```python
from build123d import *

# Parameters (mm, degrees)
SKETCH1_R           = 2.2
SKETCH1_R_2         = 0.75
BOSS_EXTRUDE1_DEPTH = 4.5
SKETCH1_3_R         = 0.75
BOSS_EXTRUDE2_DEPTH = 30


with BuildPart() as part:
    # Sketch1 → Boss-Extrude1 (new body)
    with BuildSketch(Plane(origin=(-110.040337845, 0, 0), x_dir=(0, 0, -1), z_dir=(1, 0, 0))):
        with BuildLine():
            Line((219.791431391, 54.406766631), (219.791431391, 56.131766631))
            ThreePointArc((219.791431391, 56.131766631), (219.498538172, 56.838873413), (218.791431391, 57.131766631))
            Line((218.791431391, 57.131766631), (213.191431391, 57.131766631))
            Line((213.191431391, 57.131766631), (213.191431391, 48.731766631))
            Line((213.191431391, 48.731766631), (219.791431391, 48.731766631))
            Line((219.791431391, 48.731766631), (219.791431391, 52.056766631))
            Line((219.791431391, 52.056766631), (219.351370906, 52.056766631))
            ThreePointArc((219.351370906, 52.056766631), (215.291431391, 53.231766631), (219.351370906, 54.406766631))
            Line((219.351370906, 54.406766631), (219.791431391, 54.406766631))
        make_face()
        with BuildLine():
            Line((219.791431391, 48.731766631), (213.191431391, 48.731766631))
            Line((213.191431391, 48.731766631), (213.191431391, 38.831766631))
            Line((213.191431391, 38.831766631), (218.291431391, 38.831766631))
            ThreePointArc((218.291431391, 38.831766631), (219.352091563, 39.27110646), (219.791431391, 40.331766631))
            Line((219.791431391, 40.331766631), (219.791431391, 48.731766631))
        make_face()
        with Locations((217.491431391, 42.731766631)):
            Circle(SKETCH1_R, mode=Mode.SUBTRACT)
        with BuildLine():
            Line((162.791431391, 64.577419509), (162.791431391, 55.557459873))
            ThreePointArc((162.791431391, 55.557459873), (163.541431391, 56.307459873), (164.291431391, 55.557459873))
            ThreePointArc((164.291431391, 55.557459873), (164.071761481, 55.027129792), (163.541431403, 54.807459873))
            Line((163.541431403, 54.807459873), (165.491431391, 54.807459873))
            Line((165.491431391, 54.807459873), (165.491431391, 57.431766631))
            Line((165.491431391, 57.431766631), (172.391431391, 57.431766631))
            Line((172.391431391, 57.431766631), (172.391431391, 58.231766631))
            Line((172.391431391, 58.231766631), (213.191431391, 58.231766631))
            Line((213.191431391, 58.231766631), (213.191431391, 57.431766631))
            Line((213.191431391, 57.431766631), (219.791431391, 57.431766631))
            Line((219.791431391, 57.431766631), (219.791431391, 60.200456158))
            Line((219.791431391, 60.200456158), (162.791431391, 64.577419509))
        make_face()
        with BuildLine():
            Line((219.791431391, 56.131766631), (219.791431391, 57.431766631))
            Line((219.791431391, 57.431766631), (213.191431391, 57.431766631))
            Line((213.191431391, 57.431766631), (213.191431391, 57.131766631))
            Line((213.191431391, 57.131766631), (218.791431391, 57.131766631))
            ThreePointArc((218.791431391, 57.131766631), (219.498538172, 56.838873413), (219.791431391, 56.131766631))
        make_face()
        with BuildLine():
            Line((163.541431403, 54.807459873), (162.791431391, 54.807459873))
            Line((162.791431391, 54.807459873), (162.791431391, 42.831766631))
            ThreePointArc((162.791431391, 42.831766631), (163.963004266, 40.003339507), (166.791431391, 38.831766631))
            Line((166.791431391, 38.831766631), (172.391431391, 38.831766631))
            Line((172.391431391, 38.831766631), (172.391431391, 57.431766631))
            Line((172.391431391, 57.431766631), (165.491431391, 57.431766631))
            Line((165.491431391, 57.431766631), (165.491431391, 54.807459873))
            Line((165.491431391, 54.807459873), (163.541431403, 54.807459873))
        make_face()
        with Locations((168.091431391, 42.731766631)):
            Circle(SKETCH1_R, mode=Mode.SUBTRACT)
        with Locations((168.091431391, 53.231766631)):
            Circle(SKETCH1_R, mode=Mode.SUBTRACT)
        with Locations((163.541431391, 55.557459873)):
            Circle(SKETCH1_R_2)
        with BuildLine():
            Line((162.791431391, 55.557459873), (162.791431391, 54.807459873))
            Line((162.791431391, 54.807459873), (163.541431403, 54.807459873))
            ThreePointArc((163.541431403, 54.807459873), (163.011101309, 55.027129783), (162.791431391, 55.557459873))
        make_face()
    extrude(amount=BOSS_EXTRUDE1_DEPTH)

    # Sketch1_3 → Boss-Extrude2 (add)
    with BuildSketch(Plane(origin=(-110.040337845, 0, 0), x_dir=(0, 0, -1), z_dir=(1, 0, 0))):
        with BuildLine():
            Line((162.791431391, 64.577419509), (162.791431391, 55.557459873))
            ThreePointArc((162.791431391, 55.557459873), (163.541431391, 56.307459873), (164.291431391, 55.557459873))
            ThreePointArc((164.291431391, 55.557459873), (164.071761481, 55.027129792), (163.541431403, 54.807459873))
            Line((163.541431403, 54.807459873), (165.491431391, 54.807459873))
            Line((165.491431391, 54.807459873), (165.491431391, 57.431766631))
            Line((165.491431391, 57.431766631), (172.391431391, 57.431766631))
            Line((172.391431391, 57.431766631), (172.391431391, 58.231766631))
            Line((172.391431391, 58.231766631), (213.191431391, 58.231766631))
            Line((213.191431391, 58.231766631), (213.191431391, 57.431766631))
            Line((213.191431391, 57.431766631), (219.791431391, 57.431766631))
            Line((219.791431391, 57.431766631), (219.791431391, 60.200456158))
            Line((219.791431391, 60.200456158), (162.791431391, 64.577419509))
        make_face()
        with Locations((163.541431391, 55.557459873)):
            Circle(SKETCH1_3_R)
    extrude(amount=-BOSS_EXTRUDE2_DEPTH)


solid = part.part
```
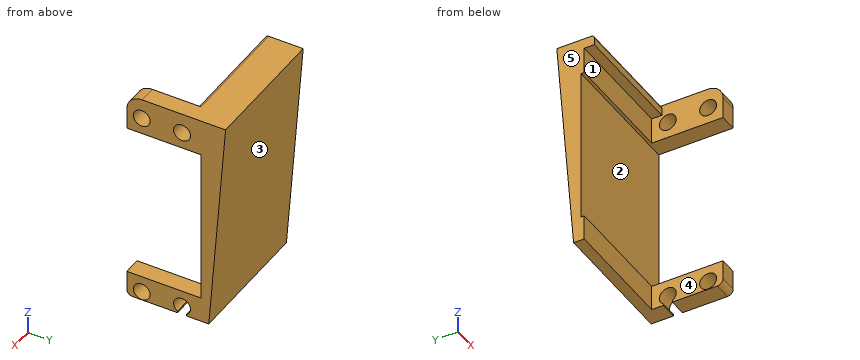
Model file for the job. Use its own axes, mm. Face numbers are marked on the shaded views. A direction names the side the tool comes from. Round coordinates to 2 decimals unless told otherwise and drop trailing zeros. Order: outer loops, then holes, each group sorted by start corner. A loop starts at its lowest first (then second) coordinate and runs counter-clockwise, first axis right, second up. Notation, with made-up numbers: M 47,-3 L 99,-3 A31 ccw 99,21 Z; hole C 62.5,-10 d10. An arc over 180 degrees is marked long. Use CSV: the item, a comma, the result in double quotes.
Item 1: Saw through at A-A (y = 42). List the corners of the cut face in (x, z), plus the area to 3 significant figures.
Worked answers:
outline,"M -110.04,-219.79 L -105.54,-219.79 L -105.54,-219.57 L -110.04,-219.57 Z; M -110.04,-215.42 L -105.54,-215.42 L -105.54,-213.19 L -110.04,-213.19 Z; M -110.04,-172.39 L -105.54,-172.39 L -105.54,-170.17 L -110.04,-170.17 Z; M -110.04,-166.02 L -105.54,-166.02 L -105.54,-162.88 L -110.04,-162.88 Z"
area,"35.2 mm²"
Item 2: Saw through at C-C (x = -116.5). List the corners of the cut face in (y, z).
Worked answers:
outline,"M 54.81,-165.49 L 57.43,-165.49 L 57.43,-172.39 L 58.23,-172.39 L 58.23,-213.19 L 57.43,-213.19 L 57.43,-219.79 L 60.2,-219.79 L 64.58,-162.79 L 55.56,-162.79 A0.75 ccw 54.81,-163.54 Z"
Item 3: Pull direction Z, two halves, no side cores. Call the marked faces 1, 2 and 3: released by +Z, released by -Z, zero draft, split by the parting line, or undercut.
Worked answers:
face 1,"zero draft"
face 2,"undercut"
face 3,"released by -Z"
Item 4: Probe probe 1 along Z at (x, y) = (-127, 55.5); probe 2 along Y at (x, z) = (-112, -214); probe 3 along Y at (x, z) = (-135, -179). List the from-to ranges inside material, lowest first.
Worked answers:
probe 1,"-165.49 to -162.79"
probe 2,"57.43 to 60.65"
probe 3,"58.23 to 63.33"
Item 5: Pin check, flat tips, straight feed: pin 1 (1 mm diameter, centred on x = -132.5, z = -164.5, fed in from -Y); pin 2 (12 mm diameter, centred on x = -116, z = -191.5, fed in from -Y); pin 3 (5 mm diameter, centred on y = 53.23, z = -168.09, fed in from -X). Stop position of each tip, or through.
Worked answers:
pin 1,"y = 54.81"
pin 2,"y = 58.23"
pin 3,"x = -110.04"
Item 6: Saw through at D-D (x = -108). List the corners of the cut face in (y, z).
Worked answers:
outline,"M 38.83,-218.29 A1.5 ccw 40.33,-219.79 L 52.06,-219.79 L 52.06,-219.35 A2.2 cw long 54.41,-219.35 L 54.41,-219.79 L 60.2,-219.79 L 64.58,-162.79 L 42.83,-162.79 A4 ccw 38.83,-166.79 L 38.83,-172.39 L 58.23,-172.39 L 58.23,-213.19 L 38.83,-213.19 Z; hole C 42.73,-217.49 d4.4; hole C 42.73,-168.09 d4.4; hole C 53.23,-168.09 d4.4"
Item 7: Saw through at B-B (z = -168). List the corners of the cut face in (x, y).
Worked answers:
outline,"M -140.04,57.43 L -110.04,57.43 L -110.04,55.43 L -105.54,55.43 L -105.54,64.18 L -140.04,64.18 Z; M -110.04,38.83 L -105.54,38.83 L -105.54,40.53 L -110.04,40.53 Z; M -110.04,44.93 L -105.54,44.93 L -105.54,51.03 L -110.04,51.03 Z"
Item 8: Which spindle directions (+Z, -Z, +X, -X, +Y, -Y) get a long thin tool onto all of the face, cutting with end or side? Do the marked faces 4 and 5. Say none if no direction does.
Worked answers:
face 4,"-Z, -X, -Y"
face 5,"+Z, -Z, -X, +Y, -Y"
